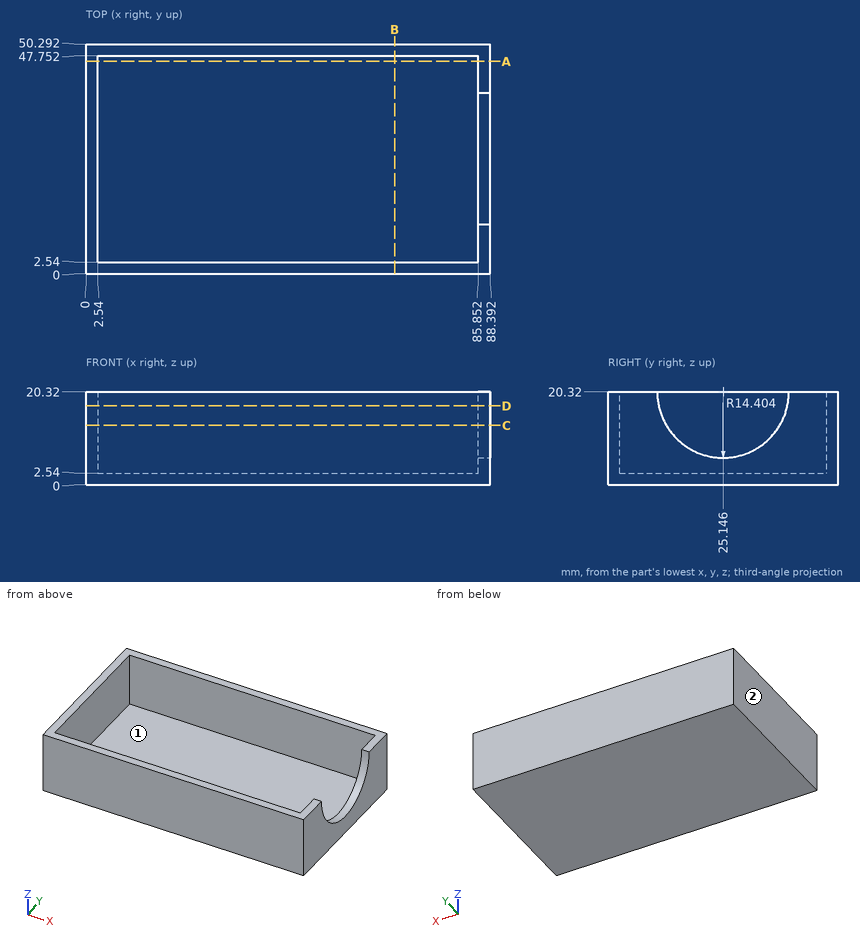
Geometry check sheet. Reference: drawing and pictorial views, mm from the part's lowest x, y, z. A direction names the side the tool comes from. Coordinates: 2 decimals unless noted, no trailing zeros. Write each loop counter-clockwise with the first axis right and the second up, starting at its lowest first coordinate (ties: lowest second). Pieces come first, ordered by that corner, then holes. Notation, with made-up numbers: (8, -26) - (19, -26) arc R27 ccw to (19, 4) - close; hole circle Ø4 at (33, 8). An arc over 180 degrees is marked (long way). One line per question, with ' | ' between items. Start each with the question number.
1. Gauge pin test, flat end, axial feed: P1, Ø5, axis at y = 22.5, z = 16.5, coming from the +X side. Record the tip position at first contact, or that the pin passes through.
2. Access from +Z, -Z, +X, -X, +Y, -Y to the whole of each face (thin tool, end or side, straight path). Record for the marked faces 1 and 2.
3. Section check B-B (x = 67.5). Enter the section's corners in (y, z).
4. Section check D-D (z = 17.25). Enter the section's corners in (x, y).
5. Section check A-A (y = 46.5). Enter the section's corners in (x, z), plus the area to 3 significant figures.
6. Section check C-C (z = 13). Enter the section's corners in (x, y).
7. Material ranges on line 1 along X through (y, z) = (7.5, 16.5); line 2 along Y through (x, z) = (75, 17); line 3 along X through (y, z) = (33, 15.75), recorded low to high.
Computed values:
1) P1: x = 2.54
2) face 1: +Z | face 2: +Z, -Z, -X, +Y, -Y
3) outline: (0, 0) - (50.29, 0) - (50.29, 20.32) - (47.75, 20.32) - (47.75, 2.54) - (2.54, 2.54) - (2.54, 20.32) - (0, 20.32) - close
4) outline: (0, 0) - (88.39, 0) - (88.39, 11.07) - (85.85, 11.07) - (85.85, 2.54) - (2.54, 2.54) - (2.54, 47.75) - (85.85, 47.75) - (85.85, 39.22) - (88.39, 39.22) - (88.39, 50.29) - (0, 50.29) - close
5) outline: (0, 0) - (88.39, 0) - (88.39, 20.32) - (85.85, 20.32) - (85.85, 2.54) - (2.54, 2.54) - (2.54, 20.32) - (0, 20.32) - close | area: 315 mm²
6) outline: (0, 0) - (88.39, 0) - (88.39, 12.74) - (85.85, 12.74) - (85.85, 2.54) - (2.54, 2.54) - (2.54, 47.75) - (85.85, 47.75) - (85.85, 37.55) - (88.39, 37.55) - (88.39, 50.29) - (0, 50.29) - close
7) line 1: 0 to 2.54, 85.85 to 88.39 | line 2: 0 to 2.54, 47.75 to 50.29 | line 3: 0 to 2.54
